Build history of the part. All positions in model axes, mm. A direction names the side the tool comes from. Give positions to 0.01 mm unless a question says otherwise; leave off trailing zeros. Order: outer loops, then holes, each group sorted by start corner. A loop starts at its lowest first (then second) coordinate and runs counter-clockwise, first axis right, second up. Notation, with made-up numbers: (81.25, 15) -> (123.25, 15) arc R22 ccw to (123.25, 34) -> close; hole circle Ø3 at (-36.75, 35). An arc over 180 degrees is marked (long way). Write item = value, one per line. Start each with the question number.
Autodesk Inventor part; units mm, degrees
ref_plane "YZ Plane" through (0, 0, 0) normal (1, 0, 0) x (0, 1, 0)
ref_plane "XZ Plane" through (0, 0, 0) normal (0, 1, 0) x (-1, 0, 0)
ref_plane "XY Plane" through (0, 0, 0) normal (0, 0, 1) x (1, 0, 0)
sketch "Sketch1" plane through (0, 0, 0) normal (0, 0, 1) x (1, 0, 0)
  line L0 (0, 0) -> (-50, 0)
  line L1 (-50, 0) -> (-50, 70)
  line L2 (-50, 70) -> (0, 70)
  line L3 (0, 70) -> (0, 0)
  dimension "d0" = 50
  dimension "d1" = 70
extrude "Extrusion1" add sketch "Sketch1" against normal blind 30
sketch "Sketch2" plane through (0, 0, 0) normal (0, 0, 1) x (1, 0, 0)
  circle A0 centre (-41.2091, 65.6547) radius 2.5
  line L0 (-41.2091, 65.6547) -> (-12.3103, 65.6547)
  circle A1 centre (-25.9431, 65.6547) radius 2.5
  circle A2 centre (-12.8739, 65.6547) radius 2.5
  circle A3 centre (-36.4759, 45.7872) radius 2.5
  line L1 (-36.4759, 45.7872) -> (-11.1478, 45.7872)
  circle A4 centre (-16.3262, 45.7872) radius 2.5
  point P0 (0, 0)
  dimension "d4" = 5
  dimension "d5" = 5
  dimension "d6" = 5
  dimension "d7" = 5
  dimension "d8" = 5
extrude "Extrusion2" add sketch "Sketch2" along normal blind 2
properties part number "subsystem1"
(1) Mould opens along Y. For faces 3 (the face through (-25, 70, -15)), 4 (the face through (-16.868, 48.228, 0.986)), 5 (the face through (-13.4, 68.1, 1)), 6 (the face through (-25, 35, -30)) say: released by +Y, released by -Y, zero draft, split by the parting line, or undercut.
(2) Cut at A-A, the plane y = 23.5. Give the cut face in (x, z), plus the area to 3 significant figures.
(3) 3-axis set-ups, long thin cutter, end or side, ignore diameter. For faces 1 (the face through (-37, 46, 2)), 2 (the face through (-41.751, 68.095, 0.986)): which of +Z, -Z, +X, -X, +Y, -Y reach the whole face in a straight line?
(4) Cut at D-D, the plane x = -40. Give the cut face in (y, z), plus the area to 3 significant figures.
(5) Cut at B-B, the plane x = -7. Give the cut face in (y, z).
(6) Cut at C-C, the plane x = -18. Give the cut face in (y, z), plus the area to 3 significant figures.
(7) Wall check: line 1 (Z direction, x = -39.5, y = 4.5). Give the ranges that are in metal, low to high. Write a range as [from, to].
(8) Flat gauge pin, fed straight in: P1, Ø8, axis at x = -32.5, y = 22, coming from the +Z side. Where does the tip first touch, or does it go through?
Results:
q1.face_3 = released by +Y
q1.face_4 = undercut
q1.face_5 = undercut
q1.face_6 = zero draft
q2.outline = (-50, -30) -> (0, -30) -> (0, 0) -> (-50, 0) -> close
q2.area = 1,500 mm2
q3.face_1 = +Z, +X, -X, +Y, -Y
q3.face_2 = +Z
q4.outline = (0, -30) -> (70, -30) -> (70, 0) -> (67.84, 0) -> (67.84, 2) -> (63.47, 2) -> (63.47, 0) -> (0, 0) -> close
q4.area = 2,110 mm2
q5.outline = (0, -30) -> (70, -30) -> (70, 0) -> (0, 0) -> close
q6.outline = (0, -30) -> (70, -30) -> (70, 0) -> (47.64, 0) -> (47.64, 2) -> (43.93, 2) -> (43.93, 0) -> (0, 0) -> close
q6.area = 2,110 mm2
q7.line_1 = [-30, 0]
q8.P1 = 0
